Autodesk Inventor part; units mm, degrees
ref_plane "YZ Plane" through (0, 0, 0) normal (1, 0, 0) x (0, 1, 0)
ref_plane "XZ Plane" through (0, 0, 0) normal (0, 1, 0) x (-1, 0, 0)
ref_plane "XY Plane" through (0, 0, 0) normal (0, 0, 1) x (1, 0, 0)
sketch "Эскиз1" plane through (0, 0, 0) normal (0, 0, 1) x (1, 0, 0)
  arc A0 (0, -35) -> (0, 35) centre (0, 0) ccw
  arc A1 (0, -45) -> (0, 45) centre (0, 0) ccw
  line L0 (0, 45) -> (0, 35)
  line L1 (0, -45) -> (0, -35)
  line L2 (0, -63) -> (0, 63)
  dimension "d0" = 35
  dimension "d1" = 45
revolve "Вращение1" add sketch "Эскиз1" angle 360 about axis through (0, -10, 0) along (0, 1, 0) contours A0 L0 A1 L1
sketch "Эскиз2" plane through (0, 0, 0) normal (0, 0, 1) x (1, 0, 0)
  circle A0 centre (0, 0) radius 10
  dimension "d3" = 20
extrude "Выдавливание1" cut sketch "Эскиз2" along normal through all
sketch "Эскиз3" plane through (0, 0, 0) normal (0, 1, 0) x (-1, 0, 0)
  line L0 (10, -45) -> (-20, -45)
  line L1 (-20, -45) -> (-20, -10)
  line L2 (-20, -10) -> (10, -10)
  line L3 (10, -10) -> (10, -45)
  line L4 (-10, 43.8748) -> (10, 43.8748)
  line L5 (-10, 43.8748) -> (10, 43.8748)
  arc A0 (-10, 43.8748) -> (10, 43.8748) centre (0, 0) ccw
  arc A1 (-10, 43.8748) -> (10, 43.8748) centre (0, 0) ccw
  dimension "d6" = 30
  dimension "d7" = 10
  dimension "d8" = 10
extrude "Выдавливание2" cut sketch "Эскиз3" along normal through all both and the other way through all contours L0 A0 L3 | L0 L1 A0 | A0 L1 L2 L3
properties part number "Нар"
Verification items for the finished model (mm, model axes). A direction names the side the tool comes from. Give positions to 0.01 mm unless a question says otherwise; leave off trailing zeros. Order: outer loops, then holes, each group sorted by start corner. A loop starts at its lowest first (then second) coordinate and runs counter-clockwise, first axis right, second up. Notation, with made-up numbers: (16, -5) -> (64, -5) arc R26 ccw to (64, 24) -> close; hole circle Ø11 at (23, 67). An arc over 180 degrees is marked (long way). Answer as CSV lines item,"result".
Q1. Sectioned sample at A-A on y = -2. Record the cut outline in (x, z).
Solutions:
outline,"(-10, -43.83) -> (-10, -33.48) arc R34.94 cw to (-9.8, 33.54) -> (-9.8, 43.87) arc R44.96 ccw to start; (9.8, 33.54) arc R34.94 cw to (20, -28.65) -> (20, -40.26) arc R44.96 ccw to (9.8, 43.87) -> close"
Q2. Sectioned sample at B-B on x = 0. Record the cut outline in (y, z), plus the area to 3 significant figures.
Solutions:
outline,"(-43.87, -10) -> (-33.54, -10) arc R35 cw to (-10, 33.54) -> (-10, 43.87) arc R45 ccw to start; (10, 33.54) arc R35 cw to (33.54, -10) -> (43.87, -10) arc R45 ccw to (10, 43.87) -> close"
area,"1,260 mm²"
Q3. Sectioned sample at C-C on z = 1.5. Record the cut outline in (x, y) (3 decimals), plus the area to 3 significant figures.
Solutions:
outline,"circle Ø89.95 at (0, 0); hole circle Ø69.936 at (0, 0)"
area,"2,510 mm²"
Q4. Depth check by flat-ended pin: pin 1 (5 mm diameter, centred on x = 25, z = 10.5, fed in from -Y); pin 2 (8 mm diameter, centred on y = 21, z = -12, fed in from -X); pin 3 (12 mm diameter, centred on x = 24, y = 12, fed in from +Z). Enter the tip coordinate at first touch or a pass-through.
Solutions:
pin 1,"stops at y = -37.67"
pin 2,"stops at x = -40.22"
pin 3,"stops at z = 39.89"
Q5. Scan lines: probe 1 along Y at (x, z) = (0, 41); probe 2 along Y at (x, z) = (7.5, 3.5); probe 3 along X at (y, z) = (0, 37). Record each from-to range of solid material in increasing order.
Solutions:
probe 1,"y = -18.55 to -10, 10 to 18.55"
probe 2,"y = -44.23 to -34.01, 34.01 to 44.23"
probe 3,"x = -25.61 to -10, 10 to 25.61"
Q6. Sectioned sample at D-D on y = 30. Record the cut outline in (x, z).
Solutions:
outline,"(-10, -32.02) -> (-10, -15) arc R18.03 cw (long way) to (15, -10) -> (20, -10) -> (20, -26.93) arc R33.54 ccw (long way) to start"
Q7. Access from +Z, -Z, +X, -X, +Y, -Y to the whole of each face (thin tool, end or side, straight path). Record for faces 1 (the flat face through (-10, -1, -34)), 2 (the cylindrical face through (-2.17, 9.76, 38.64)).
Solutions:
face 1,"-Z, +Y, -Y"
face 2,"+Z, -Z"
